Source: CAD feature listing. Evaluate the final solid. Frame: model axes, mm. Face numbers are marked on the shaded views. A direction names the side the tool comes from. Give positions to 0.01 mm unless a question says otherwise; leave off trailing zeros. Loops run counter-clockwise (first coordinate to the right, second up) from the corner with the lowest first, then second, coordinate; pieces in that order, holes last. Notation, with made-up numbers: (38, 19.25) -> (44, 19.25) arc R18 ccw to (44, 49.25) -> close; hole circle Ø7 at (-35.5, -16.75). An arc over 180 degrees is marked (long way). Return JSON: item names as keys, results as strings. Group by question number.
(1) Ray query, line 1 (X direction, y = -31.5, z = -5.5); line 2 (Z direction, x = 79, y = -54.5); line 3 (Y direction, x = 94, z = 2). Return the intervals inside material, ascending. Write a range as from..to.
(2) Pin query (flat end, axial travel): pin 1 (1.5 mm diameter, centred on x = 52.5, z = -9, fed in from +Y) (3 decimals); pin 2 (5.5 mm diameter, centred on x = 50, z = -17, fed in from -Y); pin 3 (5.5 mm diameter, centred on y = -47.5, z = 2, fed in from -X). Return the tip coordinate at first contact, or that it passes through.
(3) Cut plane B-B on z = 1.5. Return loops of the section in (x, y), then the cut area to 3 significant figures.
(4) Cut plane C-C on x = 49. Return loops of the section in (y, z).
(5) Access query for the marked faces 1 and 2. Directions: +Z, -Z, +X, -X, +Y, -Y. A direction counts if a zero-diameter tool reaches every point of the face in a straight line with its end or side. Return the directions, or none.
(6) Cut plane D-D on y = -21. Return loops of the section in (x, z), then the cut area to 3 significant figures.
(7) Cut plane A-A on x = 31. Return loops of the section in (y, z), then the cut area to 3 significant figures.
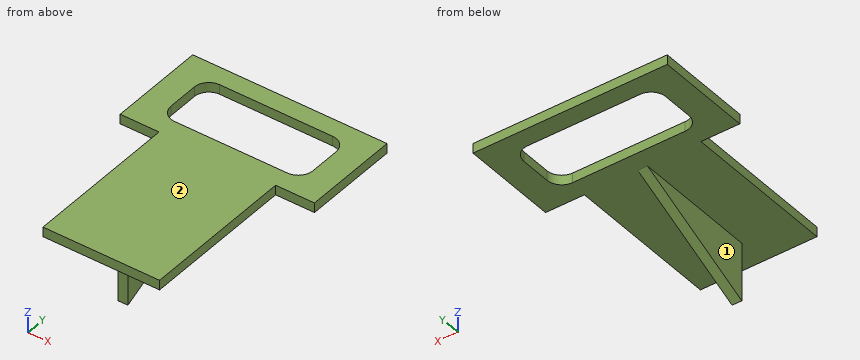
```python
from build123d import *

# Parameters (mm, degrees)
SKETCH1_W           = 100
SKETCH1_H           = 50
BOSS_EXTRUDE1_DEPTH = 5
CUT_EXTRUDE1_DEPTH  = 5
SKETCH3_W           = 60
SKETCH3_H           = 5
BOSS_EXTRUDE2_DEPTH = 80
SKETCH6_W           = 5
SKETCH6_H           = 65
BOSS_EXTRUDE4_DEPTH = 30
CUT_EXTRUDE3_DEPTH  = 5


with BuildPart() as part:
    # Sketch1 → Boss-Extrude1 (new body)
    with BuildSketch(Plane.XY):
        with Locations((50, 25)):
            Rectangle(SKETCH1_W, SKETCH1_H)
    extrude(amount=BOSS_EXTRUDE1_DEPTH)

    # Sketch2 → Cut-Extrude1 (cut)
    with BuildSketch(Plane.XY.offset(5)):
        with BuildLine():
            Line((21, 40.5), (79, 40.5))
            ThreePointArc((79, 40.5), (84.303300859, 38.303300859), (86.5, 33))
            Line((86.5, 33), (86.5, 17))
            ThreePointArc((86.5, 17), (84.303300859, 11.696699141), (79, 9.5))
            Line((79, 9.5), (21, 9.5))
            ThreePointArc((21, 9.5), (15.696699141, 11.696699141), (13.5, 17))
            Line((13.5, 17), (13.5, 33))
            ThreePointArc((13.5, 33), (15.696699141, 38.303300859), (21, 40.5))
        make_face()
    extrude(amount=-CUT_EXTRUDE1_DEPTH, mode=Mode.SUBTRACT)

    # Sketch3 → Boss-Extrude2 (add)
    with BuildSketch(Plane.XZ):
        with Locations((50, 2.5)):
            Rectangle(SKETCH3_W, SKETCH3_H)
    extrude(amount=BOSS_EXTRUDE2_DEPTH)

    # Sketch6 → Boss-Extrude4 (add)
    with BuildSketch(Plane(origin=(0, 0, 0), x_dir=(-1, 0, 0), z_dir=(0, 0, -1))):
        with Locations((-50, -32.5)):
            Rectangle(SKETCH6_W, SKETCH6_H)
    extrude(amount=BOSS_EXTRUDE4_DEPTH)

    # Sketch7 → Cut-Extrude3 (cut)
    with BuildSketch(Plane(origin=(52.5, 0, 0), x_dir=(0, 0, -1), z_dir=(1, 0, 0))):
        Polygon((0, 0), (30, -65), (30, 0), align=None)
    extrude(amount=-CUT_EXTRUDE3_DEPTH, mode=Mode.SUBTRACT)


solid = part.part
```
Answers:
{
 "1": {"line 1": "47.5..52.5", "line 2": "0..5", "line 3": "0..50"},
 "2": {"pin 1": "y = -17.875", "pin 2": "y = -65", "pin 3": "x = 20"},
 "3": {"outline": "(0, 0) -> (20, 0) -> (20, -80) -> (80, -80) -> (80, 0) -> (100, 0) -> (100, 50) -> (0, 50) -> close; hole (13.5, 17) arc R7.5 ccw to (21, 9.5) -> (79, 9.5) arc R7.5 ccw to (86.5, 17) -> (86.5, 33) arc R7.5 ccw to (79, 40.5) -> (21, 40.5) arc R7.5 ccw to (13.5, 33) -> close", "area": "7,590 mm²"},
 "4": {"outline": "(-80, 0) -> (-65, 0) -> (-65, -30) -> (0, 0) -> (9.5, 0) -> (9.5, 5) -> (-80, 5) -> close; (40.5, 0) -> (50, 0) -> (50, 5) -> (40.5, 5) -> close"},
 "5": {"face 1": "-Z, -X, +Y, -Y", "face 2": "+Z, +X, -X, +Y, -Y"},
 "6": {"outline": "(20, 0) -> (47.5, 0) -> (47.5, -9.69) -> (52.5, -9.69) -> (52.5, 0) -> (80, 0) -> (80, 5) -> (20, 5) -> close", "area": "348 mm²"},
 "7": {"outline": "(-80, 0) -> (9.5, 0) -> (9.5, 5) -> (-80, 5) -> close; (40.5, 0) -> (50, 0) -> (50, 5) -> (40.5, 5) -> close", "area": "495 mm²"}
}
